Check sheet for the drawn part. Datum: minimum x, y, z corner. Units: mm. A direction names the side the tool comes from. Give positions to 0.01 mm unless a question says otherwise; leave off trailing zeros. Loops run counter-clockwise (first coordinate to the right, second up) from the corner with the lowest first, then second, coordinate; pieces in that order, holes last. Notation, with made-up numbers: (59, 76.25) - (90, 76.25) arc R20 cw to (90, 106.25) - close; hole circle Ø2 at (31, 18.5). An arc over 180 degrees is marked (long way). One line per item, written item: value. Start each with the question number.
1. Sectioned sample at A-A (x = 15). Record the cut outline in (y, z).
2. Gauge pin test, flat ends, axial feed: pin 1 (4 mm diameter, centred on x = 23, y = 28.04, fed in from +Z); pin 2 (5 mm diameter, centred on x = 3.5, y = 32.5, fed in from -Z); pin 3 (1 mm diameter, centred on x = 12.5, z = 19.5, fed in from +Y); pin 4 (4 mm diameter, centred on y = 27.5, z = 15.5, fed in from -X). Record the tip position at first contact, or that the pin passes through.
3. Sectioned sample at C-C (y = 20). Record the cut outline in (x, z), plus the area to 3 significant figures.
4. Sectioned sample at B-B (z = 21.75). Record the cut outline in (x, y), plus the area to 3 significant figures.
5. Sectioned sample at D-D (x = 23). Record the cut outline in (y, z).
6. Mould release check, pull along Y, two halves, no side actions. Record for the marked faces 3, 4 and 5: pulls with the +Y half, pulls with the -Y half, needs draft (parallel to the pull), parting line crosses it, or undercut.
7. Scan lines: L1, parallel to X at y = 28.5, z = 19; L2, parallel to Z at x = 28, y = 12; L3, parallel to Y at x = 7, z = 21.95 (1 decimal). Record each from-to range of solid material in increasing order. Write a range as [from, to].
8. Access from +Z, -Z, +X, -X, +Y, -Y to the whole of each face (thin tool, end or side, straight path). Record for the marked faces 1 and 2.
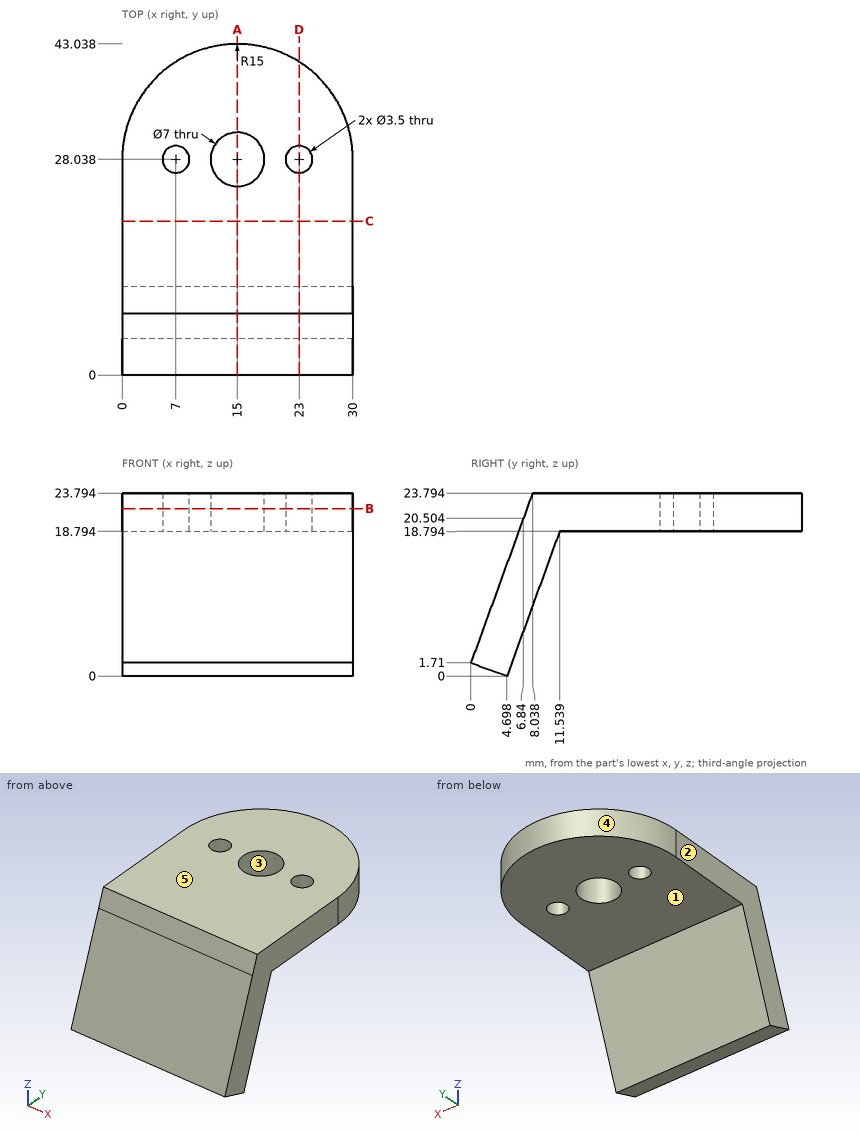
Results are:
1. outline: (0, 1.71) - (4.7, 0) - (11.54, 18.79) - (24.54, 18.79) - (24.54, 23.79) - (8.04, 23.79) - close; (31.54, 18.79) - (43.04, 18.79) - (43.04, 23.79) - (31.54, 23.79) - close
2. pin 1: stops at z = 23.79
2. pin 2: stops at z = 18.79
2. pin 3: stops at y = 42.9
2. pin 4: passes through
3. outline: (0, 18.79) - (30, 18.79) - (30, 23.79) - (0, 23.79) - close
3. area: 150 mm^2
4. outline: (0, 7.29) - (30, 7.29) - (30, 28.04) arc R15 ccw to (0, 28.04) - close; hole circle Ø3.5 at (7, 28.04); hole circle Ø7 at (15, 28.04); hole circle Ø3.5 at (23, 28.04)
4. area: 918 mm^2
5. outline: (0, 1.71) - (4.7, 0) - (11.54, 18.79) - (26.29, 18.79) - (26.29, 23.79) - (8.04, 23.79) - close; (29.79, 18.79) - (40.73, 18.79) - (40.73, 23.79) - (29.79, 23.79) - close
6. face 3: undercut
6. face 4: pulls with the +Y half
6. face 5: needs draft
7. L1: x = [0.01, 5.31], [8.69, 11.53], [18.47, 21.31], [24.69, 29.99]
7. L2: z = [18.79, 23.79]
7. L3: y = [7.4, 26.3], [29.8, 40.7]
8. face 1: -Z, +X, -X, +Y
8. face 2: +Z, -Z, -X, +Y, -Y
